CAD build for the part. Positions are in the model's coordinates, mm. A direction names the side the tool comes from. Round coordinates to 2 decimals unless told otherwise and drop trailing zeros. Order: outer loops, then holes, each group sorted by start corner. A loop starts at its lowest first (then second) coordinate and runs counter-clockwise, first axis right, second up. Notation, with made-up numbers: M -4,-19.75 L 37,-19.75 A18 cw 37,-1.75 Z; hole C 59,57 d5. An arc over 180 degrees is marked long. Answer as a JSON object with one key per item and string values.
Autodesk Inventor part; units mm, degrees
ref_plane "YZ Plane" through (0, 0, 0) normal (1, 0, 0) x (0, 1, 0)
ref_plane "XZ Plane" through (0, 0, 0) normal (0, 1, 0) x (-1, 0, 0)
ref_plane "XY Plane" through (0, 0, 0) normal (0, 0, 1) x (1, 0, 0)
sketch "スケッチ1" plane through (0, 0, 0) normal (1, 0, 0) x (0, 1, 0)
  line L0 (0, 0) -> (22, 0)
  line L1 (22, 0) -> (22, 45)
  line L2 (22, 45) -> (0, 45)
  line L3 (0, 45) -> (0, 0)
  dimension "d0" = 22
  dimension "d1" = 45
extrude "押し出し1" add sketch "スケッチ1" along normal blind 2
sketch "スケッチ2" plane through (0, 22, 45) normal (0, 1, 0) x (1, 0, 0)
  line L0 (0, 0) -> (2, 0)
  line L1 (2, 0) -> (8, 6)
  line L2 (8, 6) -> (3.3333, 10.6667)
  line L3 (3.3333, 10.6667) -> (8, 15.3333)
  line L4 (8, 15.3333) -> (3.3333, 20)
  line L5 (3.3333, 20) -> (8, 24.6667)
  line L6 (8, 24.6667) -> (3.3333, 29.3333)
  line L7 (3.3333, 29.3333) -> (8, 34)
  line L8 (8, 34) -> (2, 40)
  line L9 (2, 45) -> (2, 0)
  point P0 (0, 45)
  dimension "d4" = 40
  dimension "d5" = 6
extrude "押し出し2" add sketch "スケッチ2" against normal up to surface (22 mm away)
properties part number "finger"
Item 1: Saw through at C-C on z = 6. List the corners of the cut face in (x, y), and give its area (3 significant figures).
Worked answers:
{"outline": "M 0,0 L 3,0 L 3,22 L 0,22 Z", "area": "66.0 mm2"}
Item 2: Saw through at B-B on y = 1.5. List the corners of the cut face in (x, z).
Worked answers:
{"outline": "M 0,0 L 2,0 L 2,5 L 8,11 L 3.33,15.67 L 8,20.33 L 3.33,25 L 8,29.67 L 3.33,34.33 L 8,39 L 2,45 L 0,45 Z"}
Item 3: 3-axis set-ups, long thin cutter, end or side, ignore diameter. For faces 1 (the flat face through (1, 11, 45)), 2 (the flat face through (2, 11, 3)), 3 (the flat face through (5.699, 11.154, 27.366)): which of +Z, -Z, +X, -X, +Y, -Y reach the whole face in a straight line?
Worked answers:
{"face 1": "+Z, +X, -X, +Y, -Y", "face 2": "-Z, +X, +Y, -Y", "face 3": "+X, +Y, -Y"}
Item 4: Saw through at A-A on x = 3.75. List the corners of the cut face in (y, z), and give its area (3 significant figures).
Worked answers:
{"outline": "M 0,6.75 L 22,6.75 L 22,15.25 L 0,15.25 Z; M 0,16.08 L 22,16.08 L 22,24.58 L 0,24.58 Z; M 0,25.42 L 22,25.42 L 22,33.92 L 0,33.92 Z; M 0,34.75 L 22,34.75 L 22,43.25 L 0,43.25 Z", "area": "748 mm2"}
Item 5: Drop flat-ended pins along their axis: pin 1 Ø5.5 at (y, z) = (6.5, 2) entering from +X; pin 2 Ø1 at (x, y) = (5.5, 11.5) entering from +Z; pin 3 Ø4 at (y, z) = (5, 28) entering from +X. Give the stop position or say it passes through.
Worked answers:
{"pin 1": "stops at x = 2", "pin 2": "stops at z = 42", "pin 3": "stops at x = 8"}
Item 6: Saw through at D-D on x = 5.75. List the corners of the cut face in (y, z).
Worked answers:
{"outline": "M 0,8.75 L 22,8.75 L 22,13.25 L 0,13.25 Z; M 0,18.08 L 22,18.08 L 22,22.58 L 0,22.58 Z; M 0,27.42 L 22,27.42 L 22,31.92 L 0,31.92 Z; M 0,36.75 L 22,36.75 L 22,41.25 L 0,41.25 Z"}
Item 7: Wall check: line 1 along Z through (x, y) = (3.5, 3.5); line 2 along Z through (x, y) = (7.5, 14.25); line 3 along X through (y, z) = (20, 35). Give the ranges that are in metal, low to high. Write a range as [from, to].
Worked answers:
{"line 1": "z = [6.5, 15.5], [15.83, 24.83], [25.17, 34.17], [34.5, 43.5]", "line 2": "z = [10.5, 11.5], [19.83, 20.83], [29.17, 30.17], [38.5, 39.5]", "line 3": "x = [0, 4]"}
